Here's how the part is built. I have some questions about the finished solid (model axes, mm). Round coordinates to 2 decimals unless told otherwise and drop trailing zeros. Order: outer loops, then holes, each group sorted by start corner. A loop starts at its lowest first (then second) coordinate and runs counter-clockwise, first axis right, second up. Notation, with made-up numbers: (50.5, 66) -> (92.5, 66) arc R17 ccw to (92.5, 73) -> close; hole circle Ø4 at (-28.75, 50). An arc over 180 degrees is marked (long way). One line per item, written item: value.
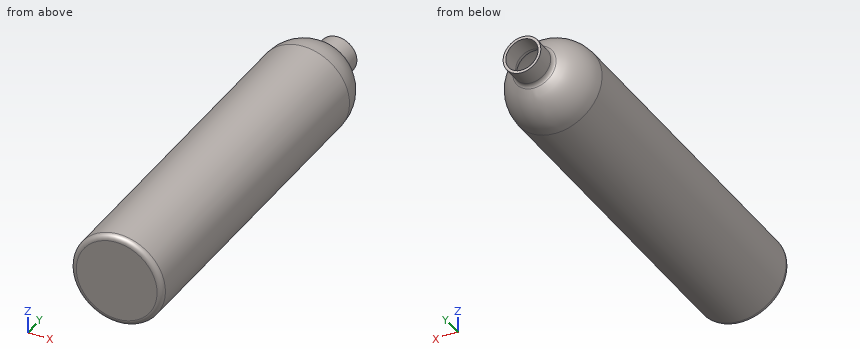
```python
from build123d import *

# Parameters (mm, degrees)
SHELL2_T = -1.5875


with BuildPart() as part:
    # Sketch4 → Revolve2 (revolve)
    with BuildSketch(Plane(origin=(0, 0, 0), x_dir=(0, 0, -1), z_dir=(1, 0, 0))):
        with BuildLine():
            Line((0, 0), (23.8125, 0))
            ThreePointArc((23.8125, 0), (26.05756403, 0.92993597), (26.9875, 3.175))
            Line((26.9875, 3.175), (26.9875, 203.2))
            ThreePointArc((26.9875, 203.2), (23.165937094, 217.044295388), (12.783552632, 226.967749964))
            ThreePointArc((12.783552632, 226.967749964), (11.562095636, 228.135215209), (11.1125, 229.763955842))
            Line((11.1125, 229.763955842), (11.1125, 240.493444248))
            Line((11.1125, 240.493444248), (0, 240.493444248))
            Line((0, 240.493444248), (0, 0))
        make_face()
    revolve(axis=Axis((0, 0, 0), (0, 1, 0)))

    # Shell2
    shell2_openings = [part.faces().sort_by_distance(p)[0] for p in [
        (0, 240.493444248, 0),
    ]]
    offset(amount=SHELL2_T, openings=shell2_openings, kind=Kind.INTERSECTION)


solid = part.part
```
Q1. For P1, Ø4, axis at x = 6, y = 29.5, coming from the -Z side; P2, Ø1.5, axis at y = 26, z = -10.5, coming from the +X side; P3, Ø6, axis at x = -8.5, y = 127, coming from the +Z side, each with a flat end and sliding along its axis, tell me the tip position at first contact or that it passes through.
Answers:
P1: z = -26.69
P2: x = 25.16
P3: z = 26.42
Q2. I want a section at C-C on y = 112.5. Write out the boundary of the cut face in (x, z) (1 decimal), then the cut area to 3 significant figures.
Answers:
outline: circle Ø54 at (0, 0); hole circle Ø50.8 at (0, 0)
area: 261 mm2
Q3. I need wall thicknesses on line 1 along X through (y, z) = (110.5, 0); line 2 along Z through (x, y) = (0, 233.75) (1 decimal). Which ranges of each line are inside material? Lowest first, please.
Answers:
line 1: -26.99 to -25.4, 25.4 to 26.99
line 2: -11.1 to -9.5, 9.5 to 11.1
